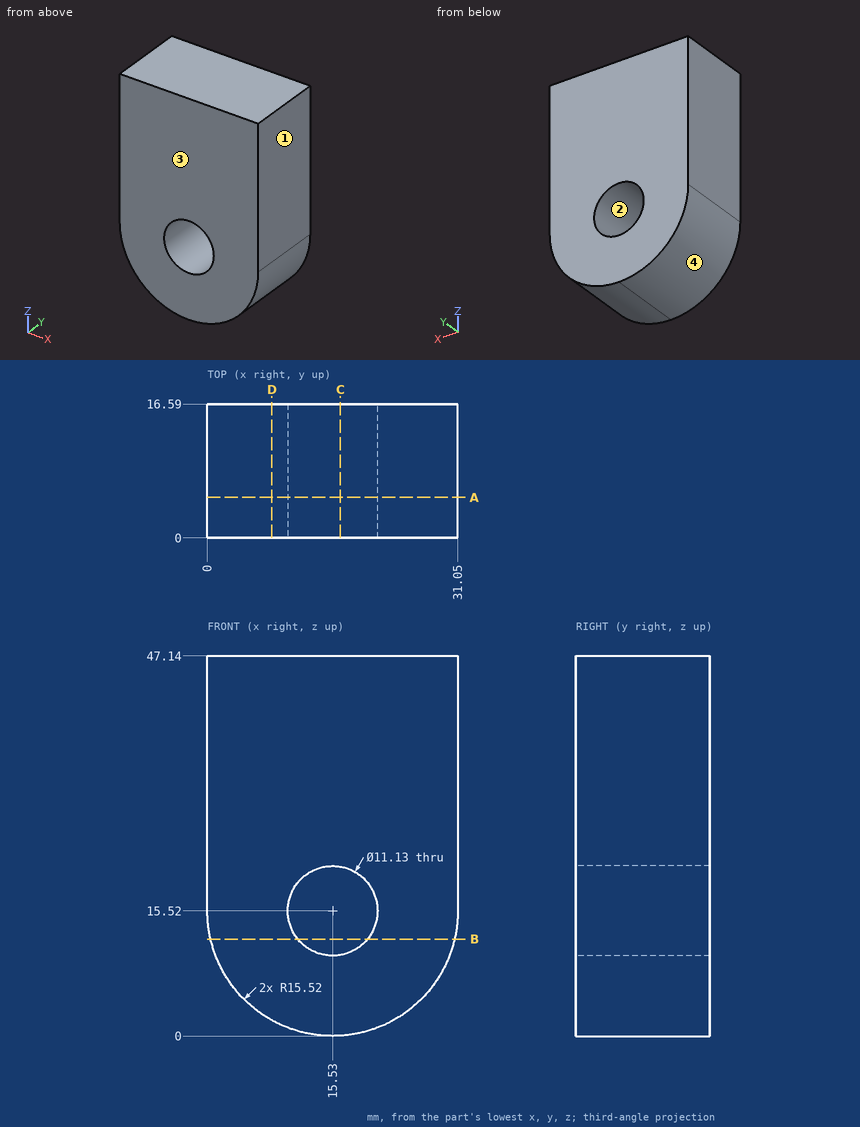
The drawing under review shows one solid part. Ordinate dimensions are in mm from its lowest x, y, z. Give positions to 0.01 mm unless a question says otherwise; leave off trailing zeros. Write each loop counter-clockwise with the first axis right and the second up, starting at its lowest first coordinate (ties: lowest second). Pieces come first, ordered by that corner, then holes. Notation, with made-up numbers: (-8, 36) -> (11, 36) arc R18 cw to (11, 42) -> close; hole circle Ø9 at (-38, 61.5). An arc over 180 degrees is marked (long way). Use CSV: the item, a comma, the result in double quotes.
Q1. Take a section at D-D, the plane x = 8. Write out the cut boundary in (y, z).
Conclusion:
outline,"(0, 1.94) -> (16.59, 1.94) -> (16.59, 47.14) -> (0, 47.14) -> close"
Q2. For P1, Ø10, axis at x = 9, z = 27.5, coming from the -Y side, flat-tipped, find the tip position at first contact; note if it passes through.
Conclusion:
P1,"y = 0"
Q3. Take a section at C-C, the plane x = 16.5. Write out the cut boundary in (y, z).
Conclusion:
outline,"(0, 0.03) -> (16.59, 0.03) -> (16.59, 10.04) -> (0, 10.04) -> close; (0, 21) -> (16.59, 21) -> (16.59, 47.14) -> (0, 47.14) -> close"
Q4. Take a section at B-B, the plane z = 12. Write out the cut boundary in (x, y).
Conclusion:
outline,"(0.4, 0) -> (11.22, 0) -> (11.22, 16.59) -> (0.4, 16.59) -> close; (19.84, 0) -> (30.65, 0) -> (30.65, 16.59) -> (19.84, 16.59) -> close"
Q5. Take a section at A-A, the plane y = 5. Write out the cut boundary in (x, z) (3 decimals), then the cut area to 3 significant figures.
Conclusion:
outline,"(0, 15.52) arc R15.52 ccw to (15.52, 0) -> (15.53, 0) arc R15.52 ccw to (31.05, 15.52) -> (31.05, 47.14) -> (0, 47.14) -> close; hole circle Ø11.13 at (15.53, 15.52)"
area,"1,260 mm2"
Q6. To check wall thickness, follow probe 1 along X at (y, z) = (4.75, 15.52) (3 decimals); probe 2 along Z at (x, y) = (13.5, 14); probe 3 along X at (y, z) = (11.25, 17). State the ranges of each line that lie inside material, in increasing order. Write a range as [from, to].
Conclusion:
probe 1,"[0, 9.965], [21.095, 31.05]"
probe 2,"[0.13, 10.34], [20.7, 47.14]"
probe 3,"[0, 10.17], [20.89, 31.05]"
Q7. Mouldability with a two-part tool opening along X and no side actions: class the marked faces 1, 2, 3 and 4 as pulls with the +X half, pulls with the -X half, needs draft (parallel to the pull), parting line crosses it, or undercut.
Conclusion:
face 1,"pulls with the +X half"
face 2,"undercut"
face 3,"needs draft"
face 4,"pulls with the -X half"
